Autodesk Inventor part; units mm, degrees
ref_plane "YZ Plane" through (0, 0, 0) normal (1, 0, 0) x (0, 1, 0)
ref_plane "XZ Plane" through (0, 0, 0) normal (0, 1, 0) x (-1, 0, 0)
ref_plane "XY Plane" through (0, 0, 0) normal (0, 0, 1) x (1, 0, 0)
sketch "Sketch1" plane through (0, 0, 0) normal (0, 0, 1) x (1, 0, 0)
  line L0 (30, 25) -> (-30, 25)
  line L1 (-30, -25) -> (-30, 25)
  line L2 (-30, -25) -> (30, -25)
  line L3 (30, 25) -> (30, -25)
  line L4 (21.9198, 18.925) -> (23.3698, 18.925)
  line L5 (23.3698, 18.925) -> (23.3698, 12.575)
  line L6 (23.3698, 12.575) -> (21.9198, 12.575)
  line L7 (21.9198, 12.575) -> (21.9198, 9.885)
  line L8 (21.9198, 9.885) -> (-2.18, 9.885)
  line L9 (-2.18, 9.885) -> (-2.18, 21.615)
  line L10 (-2.18, 21.615) -> (21.9198, 21.615)
  line L11 (21.9198, 21.615) -> (21.9198, 18.925)
  line L12 (-12.575, 23.3698) -> (-12.575, 21.9198)
  line L13 (-12.575, 21.9198) -> (-9.885, 21.9198)
  line L14 (-9.885, 21.9198) -> (-9.885, -2.18)
  line L15 (-9.885, -2.18) -> (-21.615, -2.18)
  line L16 (-21.615, -2.18) -> (-21.615, 21.9198)
  line L17 (-21.615, 21.9198) -> (-18.925, 21.9198)
  line L18 (-18.925, 21.9198) -> (-18.925, 23.3698)
  line L19 (-18.925, 23.3698) -> (-12.575, 23.3698)
  line L20 (-23.3698, -12.575) -> (-21.9198, -12.575)
  line L21 (-21.9198, -12.575) -> (-21.9198, -9.885)
  line L22 (-21.9198, -9.885) -> (2.18, -9.885)
  line L23 (2.18, -9.885) -> (2.18, -21.615)
  line L24 (2.18, -21.615) -> (-21.9198, -21.615)
  line L25 (-21.9198, -21.615) -> (-21.9198, -18.925)
  line L26 (-21.9198, -18.925) -> (-23.3698, -18.925)
  line L27 (-23.3698, -18.925) -> (-23.3698, -12.575)
  line L28 (12.575, -23.3698) -> (12.575, -21.9198)
  line L29 (12.575, -21.9198) -> (9.885, -21.9198)
  line L30 (9.885, -21.9198) -> (9.885, 2.18)
  line L31 (9.885, 2.18) -> (21.615, 2.18)
  line L32 (21.615, 2.18) -> (21.615, -21.9198)
  line L33 (21.615, -21.9198) -> (18.925, -21.9198)
  line L34 (18.925, -21.9198) -> (18.925, -23.3698)
  line L35 (18.925, -23.3698) -> (12.575, -23.3698)
  line L36 (9.885, -21.9198) -> (9.885, -25)
  line L37 (21.615, -21.9198) -> (21.615, -25)
  line L38 (-21.9198, -21.615) -> (-30, -21.615)
  line L39 (-21.9198, -9.885) -> (-30, -9.885)
  line L40 (-21.615, 21.9198) -> (-21.615, 25)
  line L41 (-9.885, 21.9198) -> (-9.885, 25)
  line L42 (21.9198, 9.885) -> (30, 9.885)
  line L43 (21.9198, 21.615) -> (30, 21.615)
  point P0 (0, 0)
extrude "Extrusion1" add sketch "Sketch1" along normal blind 2.5 contours L3 L43 L10 L9 L8 L42 L2 L37 L32 L31 L30 L36 L1 L38 L24 L23 L22 L39 L0 L40 L16 L15 L14 L41
sketch "Sketch2" plane through (0, 0, 2.5) normal (0, 0, 1) x (1, 0, 0)
  line L0 (-21.615, 25) -> (-30, 25)
  line L1 (30, -25) -> (30, 9.885)
  line L2 (-30, 25) -> (30, 25)
  line L3 (30, 25) -> (30, -25)
  line L4 (30, -25) -> (-30, -25)
  line L5 (-30, -25) -> (-30, 25)
  point P0 (0, 0)
extrude "Extrusion2" add sketch "Sketch2" along normal blind 1
properties part number "CableHolder"
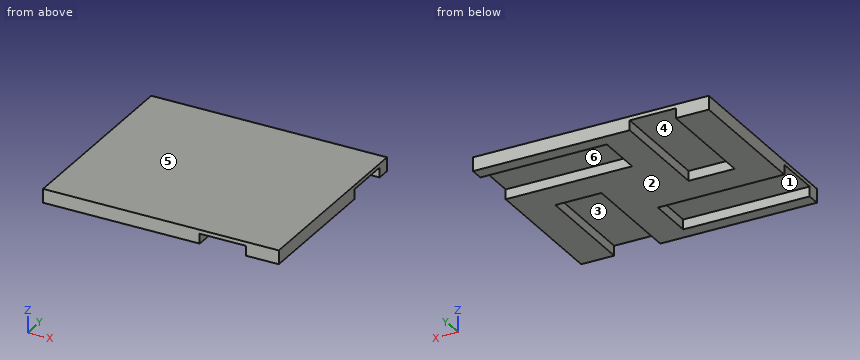
Here's how the part is built. I have some questions about the finished solid (model axes, mm). Face numbers are marked on the shaded views. A direction names the side the tool comes from. Coordinates: 2 decimals unless noted, no trailing zeros. Write each loop counter-clockwise with the first axis right and the second up, starting at its lowest first coordinate (ties: lowest second). Pieces come first, ordered by that corner, then holes. Notation, with made-up numbers: (-12, 88) -> (25, 88) arc R29 ccw to (25, 125) -> close; hole circle Ø8 at (37.25, 42.25). An arc over 180 degrees is marked (long way). Use a Markdown table: item, result. Add a question column.
(1) We'd pull the mould along Y, two halves only. Please class the marked faces 1 and 2: +Y half, -Y half, draft (parallel to the pull), parting line (faces both ways), or undercut.
(2) I'm going to push flat-ended pins straight in: P1, Ø8, axis at x = -17.5, y = 6, coming from the -Z side; P2, Ø0.8, axis at y = 17, z = 1.5, coming from the +X side; P3, Ø1.2, axis at x = 15, z = 1, coming from the -Y side; P4, Ø2, axis at x = 14, y = 1.5, coming from the -Z side. Where does each tip first touch, or does it pass through?
(3) If we section it at C-C, the plane z = 0.7: Write out the boundary of the cut face in (x, y) (3 decimals), and give its area (3 significant figures).
(4) Please list where these lines run through material, in increasing order: line 1 (Y direction, x = 1.5, z = 1.95) (3 decimals); line 2 (X direction, y = -2, z = 0.3) (3 decimals); line 3 (Y direction, x = -2.5, z = 0.45) (3 decimals).
(5) If we section it at D-D, the plane y = -4.5: Write out the boundary of the cut face in (x, z) (3 decimals), and give its area (3 significant figures).
(6) If we section it at B-B, the plane y = -12: Write out the boundary of the cut face in (x, z) (3 decimals).
(7) If we section it at A-A, the plane x = -6: Write out the boundary of the cut face in (y, z) (3 decimals).
(8) For the marked faces 3, 4, 5 and 6, which set-ups out of +Z, -Z, +X, -X, +Y, -Y let a thin tool reach every point of the face, with its end or its side?
Outcome:
| question | item | result |
|---|---|---|
| 1 | face 1 | undercut |
| 1 | face 2 | draft |
| 2 | P1 | stops at z = 2.5 |
| 2 | P2 | stops at x = -2.18 |
| 2 | P3 | stops at y = 2.18 |
| 2 | P4 | stops at z = 0 |
| 3 | outline | (-30, -25) -> (9.885, -25) -> (9.885, 2.18) -> (21.615, 2.18) -> (21.615, -25) -> (30, -25) -> (30, 9.885) -> (-2.18, 9.885) -> (-2.18, 21.615) -> (30, 21.615) -> (30, 25) -> (-9.885, 25) -> (-9.885, -2.18) -> (-21.615, -2.18) -> (-21.615, 25) -> (-30, 25) -> (-30, -9.885) -> (2.18, -9.885) -> (2.18, -21.615) -> (-30, -21.615) -> close |
| 3 | area | 1,610 mm^2 |
| 4 | line 1 | y = -25 to -21.615, -9.885 to 9.885, 21.615 to 25 |
| 4 | line 2 | x = -30 to -21.615, -9.885 to 9.885, 21.615 to 30 |
| 4 | line 3 | y = -25 to -21.615, -9.885 to 25 |
| 5 | outline | (-30, 0) -> (9.885, 0) -> (9.885, 2.5) -> (21.615, 2.5) -> (21.615, 0) -> (30, 0) -> (30, 3.5) -> (-30, 3.5) -> close |
| 5 | area | 181 mm^2 |
| 6 | outline | (-30, 2.5) -> (2.18, 2.5) -> (2.18, 0) -> (9.885, 0) -> (9.885, 2.5) -> (21.615, 2.5) -> (21.615, 0) -> (30, 0) -> (30, 3.5) -> (-30, 3.5) -> close |
| 7 | outline | (-25, 0) -> (-21.615, 0) -> (-21.615, 2.5) -> (-9.885, 2.5) -> (-9.885, 0) -> (25, 0) -> (25, 3.5) -> (-25, 3.5) -> close |
| 8 | face 3 | -Z, -Y |
| 8 | face 4 | -Z, +Y |
| 8 | face 5 | +Z, +X, -X, +Y, -Y |
| 8 | face 6 | -Z, +X |
